from build123d import *

# Parameters (mm, degrees)
BOSS_EXTRUDE1_DEPTH     = 25
CUT_EXTRUDE1_DEPTH      = 118.647905993
CUT_EXTRUDE1_DEPTH_BACK = 118.647905993
SKETCH2_R               = 4.5
SKETCH4_R               = 1
CUT_EXTRUDE3_DEPTH      = 114.903893928
SKETCH5_R               = 2.25
CUT_EXTRUDE4_DEPTH      = 13


with BuildPart() as part:
    # Sketch1 → Boss-Extrude1 (new body)
    with BuildSketch(Plane(origin=(-10, 0, 0), x_dir=(0, 0, -1), z_dir=(1, 0, 0))):
        with BuildLine():
            Line((-95.101282582, 44.173788963), (-95.219276466, 45.957628532))
            ThreePointArc((-95.219276466, 45.957628532), (-92.763433913, 53.206592673), (-85.901099289, 56.595841451))
            Line((-85.901099289, 56.595841451), (-75.922904242, 57.255859321))
            ThreePointArc((-75.922904242, 57.255859321), (-82.156438236, 45.925861069), (-74.484874616, 35.515629656))
            Line((-74.484874616, 35.515629656), (-84.463069663, 34.855611786))
            ThreePointArc((-84.463069663, 34.855611786), (-91.712033804, 37.311454339), (-95.101282582, 44.173788963))
        make_face()
    extrude(amount=BOSS_EXTRUDE1_DEPTH)

    # Sketch2 → Cut-Extrude1 (cut, two sides: drawn at the far end of the back side and taken through both)
    with BuildSketch(Plane(origin=(0, 0.216574413, -6.555528357), x_dir=(1, 0, 0), z_dir=(0, -0.06600178707669223, 0.9978195047716211)).offset(-CUT_EXTRUDE1_DEPTH_BACK)):
        with Locations(Location((5.5, 51.464766105, 0), (0, 0, 90))):
            Circle(SKETCH2_R)
    extrude(amount=CUT_EXTRUDE1_DEPTH + CUT_EXTRUDE1_DEPTH_BACK, mode=Mode.SUBTRACT)

    # Sketch4 → Cut-Extrude3 (cut, through all)
    with BuildSketch(Plane.ZY.offset(10)):
        with Locations(Location((85.669468509, 53.094031558, 0), (0, 0, 270))):
            Circle(SKETCH4_R)
        with Locations(Location((84.694700444, 38.357421678, 0), (0, 0, 270))):
            Circle(SKETCH4_R)
    extrude(amount=-CUT_EXTRUDE3_DEPTH, mode=Mode.SUBTRACT)

    # Sketch5 → Cut-Extrude4 (cut)
    with BuildSketch(Plane(origin=(15, 0, 0), x_dir=(0, 0, -1), z_dir=(1, 0, 0))):
        with Locations(Location((-84.694700444, 38.357421678, 0), (0, 0, 90))):
            Circle(SKETCH5_R)
        with Locations(Location((-85.669468509, 53.094031558, 0), (0, 0, 90))):
            Circle(SKETCH5_R)
    extrude(amount=-CUT_EXTRUDE4_DEPTH, mode=Mode.SUBTRACT)


solid = part.part
Geometry: final body of the model. Coordinates: model frame, mm. A direction names the side the tool comes from. Give positions to 0.01 mm unless a question says otherwise; leave off trailing zeros. Loops run counter-clockwise (first coordinate to the right, second up) from the corner with the lowest first, then second, coordinate; pieces in that order, holes last. Notation, with made-up numbers: (-27, 34.25) - (-20, 34.25) arc R20 ccw to (-20, 43.25) - close; hole circle Ø2 at (-17.75, 30). An arc over 180 degrees is marked (long way). Answer as CSV lines item,"result". Start each with the question number.
1. Draft query along Y for faces 1 (the face through (2.32, 56.92, 80.98)), 2 (the face through (2.32, 35.19, 79.4)), 3 (the face through (2, 53, 87)), 4 (the face through (15, 46, 87)). Return one class per face: released by +Y, released by -Y, zero draft, split by the parting line, or undercut.
2. Pin query (flat end, axial travel): P1, Ø8, axis at x = 1.5, y = 40, coming from the -Z side; P2, Ø8, axis at x = 9.5, z = 80.5, coming from the -Y side; P3, Ø6, axis at x = 10, z = 79.5, coming from the +Y side; P4, Ø1.8, axis at y = 38.36, z = 84.69, coming from the -X side. Return the tip coordinate at first contact, or that it passes through.
3. Section B-B, the plane z = 78.75. Return loops of the section in (x, y).
4. Reachability of faces 5 (the face through (-4.084, 52.556, 86.513)), 6 (the face through (2, 37, 85)) from +Z, -Z, +X, -X, +Y, -Y: full face, straight path, thin tool, end or side. Return the list, or none.
5. Ray query, L1, parallel to Y at x = 5, z = 85; L2, parallel to Y at x = -2.25, z = 85.5; L3, parallel to Z at x = -1.25, y = 53.75. Return the intervals inside material, ascending.
6. Section A-A, the plane x = 3. Return loops of the section in (y, z).
7. Section C-C, the plane x = 12. Return loops of the section in (y, z), plus the area to 3 significant figures.
8. Section D-D, the plane y = 54.5. Return loops of the section in (x, z), plus the area to 3 significant figures.
Answers:
1,face 1,"released by +Y"
1,face 2,"released by -Y"
1,face 3,"undercut"
1,face 4,"zero draft"
2,P1,"stops at z = 75.58"
2,P2,"stops at y = 34.85"
2,P3,"stops at y = 57.22"
2,P4,"passes through"
3,outline,"(-10, 35.23) - (15, 35.23) - (15, 38.32) - (-10, 38.32) - close; (-10, 55.12) - (15, 55.12) - (15, 57.07) - (-10, 57.07) - close"
4,face 5,"+X, -X"
4,face 6,"+X"
5,L1,"y = 34.83 to 36.13, 40.59 to 41.26, 50.22 to 50.95, 55.24 to 56.66"
5,L2,"y = 34.84 to 37.76, 38.95 to 52.11, 54.08 to 56.62"
5,L3,"z = 79.91 to 84.91, 86.42 to 92.25"
6,outline,"(34.86, 84.46) - (35.52, 74.48) arc R12 cw to (42.23, 81.31) - (41.36, 94.5) arc R10 ccw to start; (48.83, 94.99) - (49.7, 81.81) arc R12 cw to (57.26, 75.92) - (56.6, 85.9) arc R10 ccw to start; hole circle Ø4.5 at (38.36, 84.69); hole circle Ø4.5 at (53.09, 85.67)"
7,outline,"(34.86, 84.46) - (35.52, 74.48) arc R12 cw to (57.26, 75.92) - (56.6, 85.9) arc R10 ccw to (45.96, 95.22) - (44.17, 95.1) arc R10 ccw to start; hole circle Ø4.5 at (38.36, 84.69); hole circle Ø4.5 at (53.09, 85.67)"
7,area,"252 mm2"
8,outline,"(-10, 79.32) - (15, 79.32) - (15, 83.91) - (2, 83.91) - (2, 87.43) - (15, 87.43) - (15, 91.39) - (-10, 91.39) - close"
8,area,"256 mm2"
